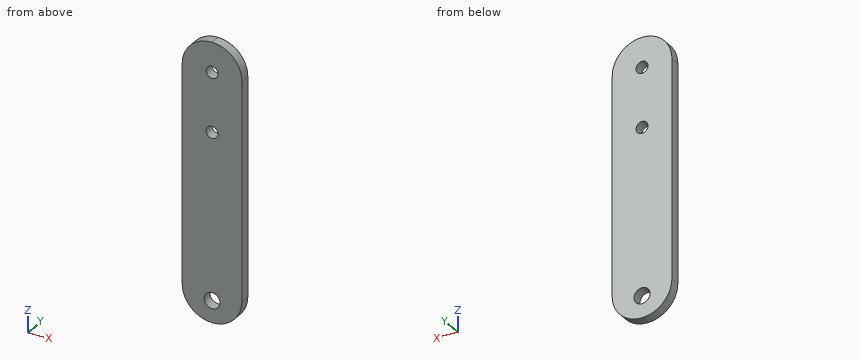
from build123d import *

# Parameters (mm, degrees)
ESQUISSE1_W      = 15
ESQUISSE1_H      = 2.5
EXTRUSION1_DEPTH = 70
CONG_1_R         = 7.5
ESQUISSE2_R      = 1.5
EXTRUSION2_DEPTH = 71.445014018
ESQUISSE3_R      = 2
EXTRUSION3_DEPTH = 71.445014018
CONG_2_R         = 7.5
ESQUISSE4_R      = 1.5
EXTRUSION4_DEPTH = 71.445014018


with BuildPart() as part:
    # Esquisse1 → Extrusion1 (new body)
    with BuildSketch(Plane.XY):
        Rectangle(ESQUISSE1_W, ESQUISSE1_H)
    extrude(amount=EXTRUSION1_DEPTH)

    # Congé1
    cong_1_edges = [part.edges().sort_by_distance(p)[0] for p in [
        (-7.5, 0, 70),
        (7.5, 0, 70),
    ]]
    fillet(cong_1_edges, radius=CONG_1_R - 0.0001)  # a hair under: the kernel refuses the full size

    # Esquisse2 → Extrusion2 (cut, through all)
    with BuildSketch(Plane(origin=(0, 1.25, 0), x_dir=(1, 0, 0), z_dir=(0, 1, 0))):
        with Locations(Location((0, -62.5, 0), (0, 0, 270))):
            Circle(ESQUISSE2_R)
    extrude(amount=-EXTRUSION2_DEPTH, mode=Mode.SUBTRACT)

    # Esquisse3 → Extrusion3 (cut, through all)
    with BuildSketch(Plane(origin=(0, 1.25, 0), x_dir=(1, 0, 0), z_dir=(0, 1, 0))):
        with Locations(Location((0, -5.5, 0), (0, 0, 270))):
            Circle(ESQUISSE3_R)
    extrude(amount=-EXTRUSION3_DEPTH, mode=Mode.SUBTRACT)

    # Congé2
    cong_2_edges = [part.edges().sort_by_distance(p)[0] for p in [
        (7.5, 0, 0),
        (-7.5, 0, 0),
    ]]
    fillet(cong_2_edges, radius=CONG_2_R - 0.0001)  # a hair under: the kernel refuses the full size

    # Esquisse4 → Extrusion4 (cut, through all)
    with BuildSketch(Plane(origin=(0, 1.25, 0), x_dir=(1, 0, 0), z_dir=(0, 1, 0))):
        with Locations(Location((0, -47.5, 0), (0, 0, 270))):
            Circle(ESQUISSE4_R)
    extrude(amount=-EXTRUSION4_DEPTH, mode=Mode.SUBTRACT)


solid = part.part
For this review, take the finished solid that the model builds, in its own axes (mm). Round coordinates to 2 decimals unless told otherwise and drop trailing zeros. Loops run counter-clockwise (first coordinate to the right, second up) from the corner with the lowest first, then second, coordinate; pieces in that order, holes last. Notation, with made-up numbers: (27.5, 32.5) - (74.5, 32.5) arc R24 cw to (74.5, 45.5) - close; hole circle Ø5 at (85.25, -4). An arc over 180 degrees is marked (long way). Use one line per item in the form item = value.
Item 1: Consider section A-A on z = 47.5. Write out the cut boundary in (x, y), then the cut area to 3 significant figures.
Answers:
outline = (-7.5, -1.25) - (-1.5, -1.25) - (-1.5, 1.25) - (-7.5, 1.25) - close; (1.5, -1.25) - (7.5, -1.25) - (7.5, 1.25) - (1.5, 1.25) - close
area = 30.0 mm^2
Item 2: Consider section B-B on y = -0.25. State how many separate pieces and enclosed holes the cut face has, then the cut area to 3 significant figures.
Answers:
separate_pieces = 1
enclosed_holes = 3
area = 975 mm^2
Item 3: For line 1 (X direction, y = -0.15, z = 62.5); line 2 (Z direction, x = -1.25, y = 0.8); line 3 (X direction, y = 0.35, z = 48), list the stretches that pass through material, from the lowest coordinate up.
Answers:
line_1 = -7.5 to -1.5, 1.5 to 7.5
line_2 = 0.1 to 3.94, 7.06 to 46.67, 48.33 to 61.67, 63.33 to 69.9
line_3 = -7.5 to -1.41, 1.41 to 7.5
Item 4: Consider section C-C on z = 5.5. Write out the cut boundary in (x, y).
Answers:
outline = (-7.23, -1.25) - (-2, -1.25) - (-2, 1.25) - (-7.23, 1.25) - close; (2, -1.25) - (7.23, -1.25) - (7.23, 1.25) - (2, 1.25) - close
Item 5: Clearance check with flat-ended pins moving along their axes: P1, Ø1.5, axis at x = -1, y = -1, coming from the -Z side; P2, Ø2.5, axis at x = 0, z = 47.5, coming from the +Y side. State where each tip first meets the part, or that it passes through.
Answers:
P1 = 0
P2 = through
Item 6: Consider section D-D on x = 5.75. Write out the cut boundary in (y, z), then the cut area to 3 significant figures.
Answers:
outline = (-1.25, 2.68) - (1.25, 2.68) - (1.25, 67.32) - (-1.25, 67.32) - close
area = 162 mm^2
